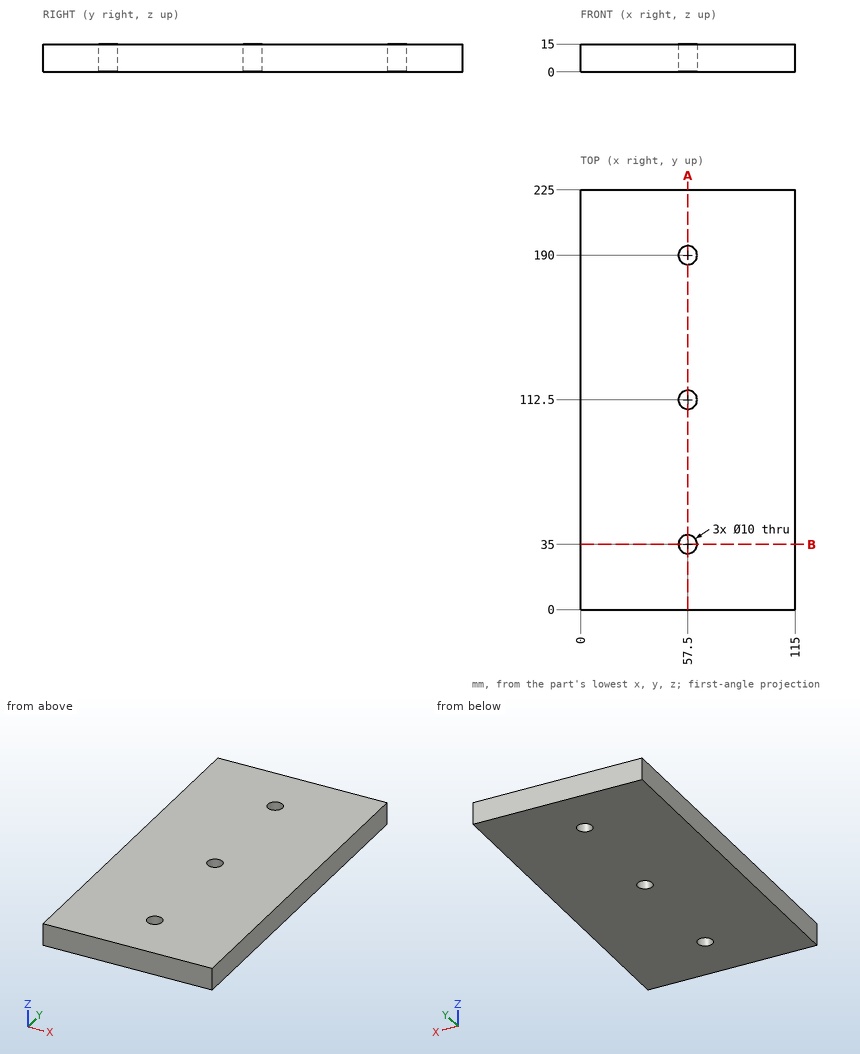
Verification items for this drawing (mm, ordinates from the low corner). Give positions to 0.01 mm unless a question says otherwise; leave off trailing zeros. Write each loop counter-clockwise with the first axis right and the second up, starting at its lowest first coordinate (ties: lowest second). Pieces come first, ordered by that corner, then holes. Notation, with made-up numbers: (36, 1.5) -> (79, 1.5) arc R20 ccw to (79, 26.5) -> close; hole circle Ø8 at (69, -11). An arc over 180 degrees is marked (long way). Use CSV: the item, a comma, the result in double quotes.
(1) Material ranges on L1, parallel to X at y = 35, z = 6.25; L2, parallel to Y at x = 57.5, z = 5; L3, parallel to X at y = 32.5, z = 8.5, recorded low to high.
Derived:
L1,"x = 0 to 52.5, 62.5 to 115"
L2,"y = 0 to 30, 40 to 107.5, 117.5 to 185, 195 to 225"
L3,"x = 0 to 53.17, 61.83 to 115"
(2) Go/stop test with flat-tipped pins: pin 1 (9 mm diameter, centred on x = 57.5, y = 35, fed in from +Z); pin 2 (6 mm diameter, centred on y = 105, z = 12.5, fed in from -X). Record where each tip stops, or that it passes through.
Derived:
pin 1,"passes through"
pin 2,"stops at x = 0"
(3) Sectioned sample at A-A (x = 57.5). Record the cut outline in (y, z), plus the area to 4 significant figures.
Derived:
outline,"(0, 0) -> (30, 0) -> (30, 15) -> (0, 15) -> close; (40, 0) -> (107.5, 0) -> (107.5, 15) -> (40, 15) -> close; (117.5, 0) -> (185, 0) -> (185, 15) -> (117.5, 15) -> close; (195, 0) -> (225, 0) -> (225, 15) -> (195, 15) -> close"
area,"2,925 mm^2"
(4) Sectioned sample at B-B (y = 35). Record the cut outline in (x, z), plus the area to 4 significant figures.
Derived:
outline,"(0, 0) -> (52.5, 0) -> (52.5, 15) -> (0, 15) -> close; (62.5, 0) -> (115, 0) -> (115, 15) -> (62.5, 15) -> close"
area,"1,575 mm^2"
